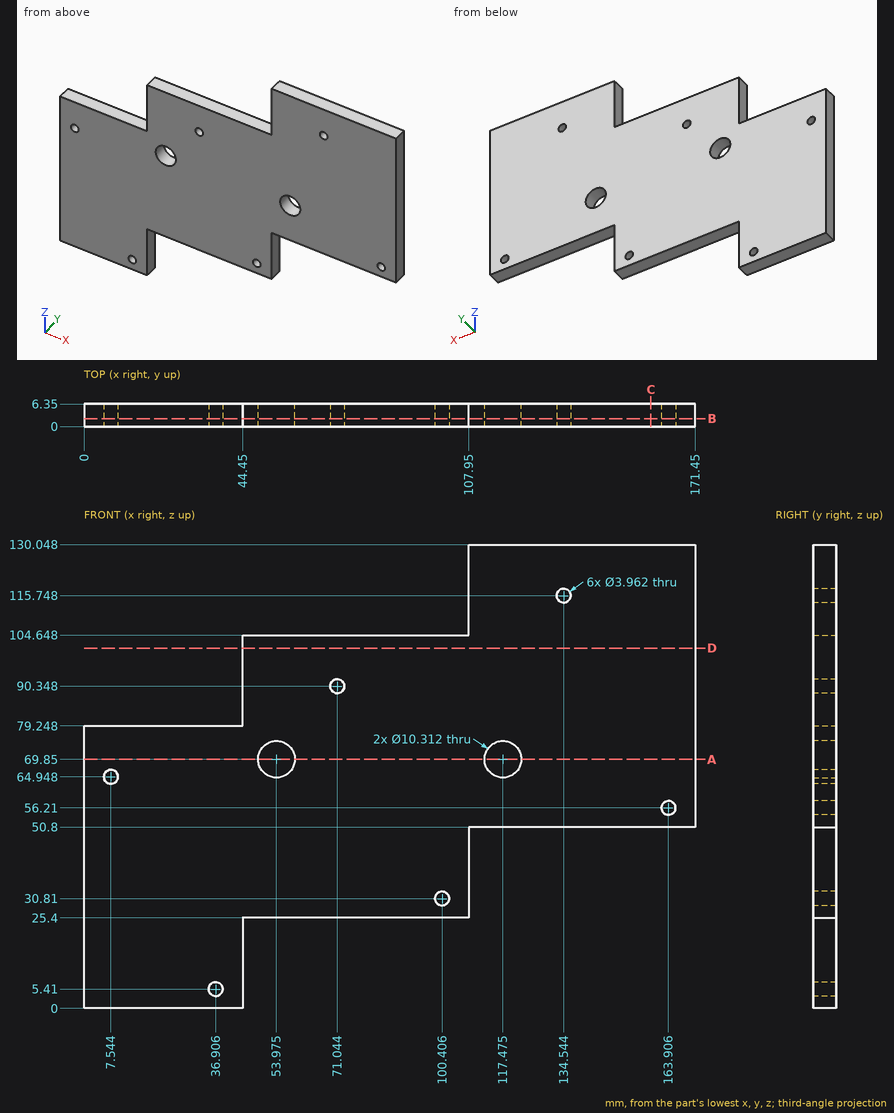
Can you work these out from the drawing? Everything is in mm from the part's minimum corner. Round coordinates to 2 decimals unless told otherwise and drop trailing zeros. Loops run counter-clockwise (first coordinate to the right, second up) from the corner with the lowest first, then second, coordinate; pieces in that order, holes last.
1. If I drill on line 1 along X through (y, z) = (4.25, 69.85); line 2 along Z through (x, y) = (11.5, 3.75); line 3 along Z through (x, y) = (151.5, 2.75), over which ranges is the centre line in solid material (lowest first)?
Answer list:
line 1: x = 0 to 48.82, 59.13 to 112.32, 122.63 to 171.45
line 2: z = 0 to 79.25
line 3: z = 50.8 to 130.05
2. For P1, Ø1.9, axis at x = 129, y = 3.5, coming from the -Z side; P2, Ø1.9, axis at y = 4.5, z = 44, coming from the +X side, each with a flat end and sliding along its axis, tell me the tip position at first contact or that it passes through.
Answer list:
P1: stops at z = 50.8
P2: stops at x = 107.95
3. If we section it at B-B on y = 2.25: Count the separate pieces of the cut face and the enclosed holes in it, plus the area to 3 significant figures.
Answer list:
separate pieces: 1
enclosed holes: 8
area: 13,300 mm2
4. If we section it at A-A on z = 69.85: Write out the boundary of the cut face in (x, y).
Answer list:
outline: (0, 0) - (48.82, 0) - (48.82, 6.35) - (0, 6.35) - close; (59.13, 0) - (112.32, 0) - (112.32, 6.35) - (59.13, 6.35) - close; (122.63, 0) - (171.45, 0) - (171.45, 6.35) - (122.63, 6.35) - close
5. If we section it at C-C on x = 159: Write out the boundary of the cut face in (y, z).
Answer list:
outline: (0, 50.8) - (6.35, 50.8) - (6.35, 130.05) - (0, 130.05) - close
6. If we section it at D-D on z = 101: Write out the boundary of the cut face in (x, y).
Answer list:
outline: (44.45, 0) - (171.45, 0) - (171.45, 6.35) - (44.45, 6.35) - close
